The model under review builds one solid part; all positions refer to its coordinate system, in mm. Face numbers are marked on the shaded views. A direction names the side the tool comes from. Round coordinates to 2 decimals unless told otherwise and drop trailing zeros. Write each loop counter-clockwise with the first axis right and the second up, starting at its lowest first coordinate (ties: lowest second). Pieces come first, ordered by that corner, then holes. Notation, with made-up numbers: (57, 37) -> (96, 37) arc R16 cw to (96, 43) -> close; hole circle Ø11 at (-30.75, 77.5). An arc over 180 degrees is marked (long way). Return JSON: item names as keys, results as strings. Group by question number.
1. Take a section at D-D, the plane z = 9.5. Write out the cut boundary in (x, y).
2. Take a section at A-A, the plane z = -9.75. Write out the cut boundary in (x, y).
3. Take a section at C-C, the plane x = -11.5. Give the number of separate pieces and of enclosed holes in the cut face, then the cut area to 3 significant figures.
4. For line 1 along Z through (x, y) = (-5.5, -14.5); line 2 along Z through (x, y) = (-6, 1.5); line 3 along X through (y, z) = (-8, 9), list the stretches that pass through material, from the lowest coordinate up. Write a range as from..to.
5. Take a section at B-B, the plane y = 6.5. Write out the cut boundary in (x, z), then the cut area to 3 significant figures.
6. Clearance check with flat-ended pins moving along their axes: P1, Ø4, axis at x = -25.5, y = 0.5, coming from the -Z side; P2, Ø4.5, axis at x = -4.5, y = -7.5, coming from the -Z side; P3, Ø3, axis at y = 12, z = 6.5, coming from the +X side. State where each tip first meets the part, or that it passes through.
7. Mouldability with a two-part tool opening along Y and no side actions: class the marked faces 4, 5 and 6 as pulls with the +Y half, pulls with the -Y half, needs draft (parallel to the pull), parting line crosses it, or undercut.
8. Tool access review of the marked faces 1, 2 and 3: name each direction out of +Z, -Z, +X, -X, +Y, -Y from which nothing blocks a thin tool from reaching the whole face with its end or side.
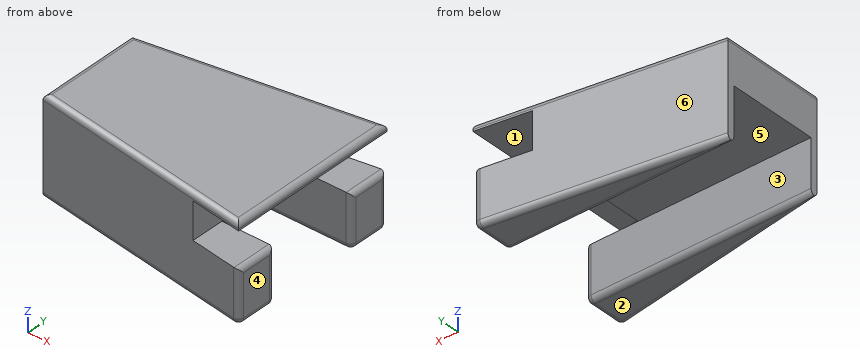
from build123d import *

# Parameters (mm, degrees)
F0_W         = 64.5
F0_H         = 13
F0_H_2       = 2
F1_DEPTH     = 12.5
F2_DEPTH     = 15
F4_DEPTH     = 15
F6_T1_DEPTH  = 72.7705906209
F6_T3_DEPTH  = 57.5
F6_T5_DEPTH  = 72.7705906209
F6_T7_DEPTH  = 37.5
F6_T9_DEPTH  = 66.75
F6_T11_DEPTH = 67.2701117692
F6_T13_DEPTH = 8.7495211484
F6_T15_DEPTH = 67.2701117692
F6_T17_DEPTH = 8.7495211484
F6_T19_DEPTH = 17.8761971291
F6_T21_DEPTH = 17.25
F6_T23_DEPTH = 19.5
F6_T25_DEPTH = 19.5
F6_S29_W     = 1.53
F6_S29_H     = 1.53
F6_T30_DEPTH = 1.53
F6_T36_DEPTH = 1.53
F6_S41_W     = 1.53
F6_S41_H     = 1.53
F6_T42_DEPTH = 1.53
F6_T48_DEPTH = 1.53
F6_T54_DEPTH = 9.5
F6_S55_R     = 1.5
F6_T56_DEPTH = 6
F6_T60_DEPTH = 9.5
F6_S61_R     = 1.5
F6_T62_DEPTH = 6
F6_T66_DEPTH = 9.5
F6_S67_R     = 1.5
F6_T68_DEPTH = 6
F6_T72_DEPTH = 9.5
F6_S73_R     = 1.5
F6_T74_DEPTH = 6


# Not quite as in the source:
# - a fillet or chamfer that OpenCascade refuses, or shapes differently, is made with other operations: its cross-section is extruded or revolved along the edge and cut away or added
# - a feature names something its author has since deleted; it is built from what else it names


with BuildPart() as f1:
    # F0 (on Top) → F1 (new body)
    with BuildSketch(Plane.XY):
        with Locations((-32.25, -6.5)):
            Rectangle(F0_W, F0_H)
        with Locations((-32.25, -14)):
            Rectangle(F0_W, F0_H_2)
        Polygon((0, -15), (-64.5, -15), (0, -25), align=None)
    extrude(amount=F1_DEPTH)

    # F0 (on Top) → F2 (join)
    with BuildSketch(Plane.XY):
        with Locations((-32.25, -14)):
            Rectangle(F0_W, F0_H_2)
        Polygon((0, -15), (-64.5, -15), (0, -25), align=None)
    extrude(amount=-F2_DEPTH)

    # F3 (on face) → F4 (cut)
    with BuildSketch(Plane.YZ):
        Polygon((-13, 0), (0, 0), (0, 10.5), (-25, 10.5), (-25, 0), align=None)
    extrude(amount=-F4_DEPTH, mode=Mode.SUBTRACT)

    # F5: F1 across plane


with BuildPart() as f1_1:
    add(f1.part)
    add(f1.part.mirror(Plane.XZ))

    # F6: fillet of radius 1.5 on 18 edges, made by hand

    # F6_s2 → F6_t1 (cut)
    with BuildSketch(Plane(origin=(-64.4207380098, 9.9877113194, 0), x_dir=(0, 0, 1), z_dir=(0.9881939076, -0.1532083578, 0))):
        with BuildLine():
            ThreePointArc((11, 24.7048476911), (12.0606601718, 24.2655078629), (12.5, 23.2048476911))
            Line((12.5, 23.2048476911), (12.5, 24.7048476911))
            Line((12.5, 24.7048476911), (11, 24.7048476911))
        make_face()
    extrude(amount=F6_T1_DEPTH, mode=Mode.SUBTRACT)

    # F6_s4 → F6_t3 (cut)
    with BuildSketch(Plane.XZ.offset(-28.75)):
        with BuildLine():
            ThreePointArc((-1.5, 12.5), (-0.4393398282, 12.0606601718), (0, 11))
            Line((0, 11), (0, 12.5))
            Line((0, 12.5), (-1.5, 12.5))
        make_face()
    extrude(amount=F6_T3_DEPTH, mode=Mode.SUBTRACT)

    # F6_s6 → F6_t5 (cut)
    with BuildSketch(Plane(origin=(-64.4207380098, -9.9877113194, 0), x_dir=(0, 0, 1), z_dir=(0.9881939076, 0.1532083578, 0))):
        with BuildLine():
            ThreePointArc((12.5, -23.2048476911), (12.0606601718, -24.2655078629), (11, -24.7048476911))
            Line((11, -24.7048476911), (12.5, -24.7048476911))
            Line((12.5, -24.7048476911), (12.5, -23.2048476911))
        make_face()
    extrude(amount=F6_T5_DEPTH, mode=Mode.SUBTRACT)

    # F6_s8 → F6_t7 (cut)
    with BuildSketch(Plane.XZ.offset(-18.75)):
        with BuildLine():
            ThreePointArc((-63, 12.5), (-64.0606601718, 12.0606601718), (-64.5, 11))
            Line((-64.5, 11), (-64.5, 12.5))
            Line((-64.5, 12.5), (-63, 12.5))
        make_face()
    extrude(amount=F6_T7_DEPTH, mode=Mode.SUBTRACT)

    # F6_s10 → F6_t9 (cut)
    with BuildSketch(Plane.YZ.offset(-68.25)):
        with BuildLine():
            ThreePointArc((-13, -13.5), (-13.4393398282, -14.5606601718), (-14.5, -15))
            Line((-14.5, -15), (-13, -15))
            Line((-13, -15), (-13, -13.5))
        make_face()
        with BuildLine():
            ThreePointArc((13, -13.5), (13.4393398282, -14.5606601718), (14.5, -15))
            Line((14.5, -15), (13, -15))
            Line((13, -15), (13, -13.5))
        make_face()
    extrude(amount=F6_T9_DEPTH, mode=Mode.SUBTRACT)

    # F6_s12 → F6_t11 (cut)
    with BuildSketch(Plane(origin=(-64.4207380098, 9.9877113194, 0), x_dir=(0, 0, 1), z_dir=(0.9881939076, -0.1532083578, 0))):
        with BuildLine():
            ThreePointArc((-13.5, 24.7048476911), (-14.5606601718, 24.2655078629), (-15, 23.2048476911))
            Line((-15, 23.2048476911), (-15, 24.7048476911))
            Line((-15, 24.7048476911), (-13.5, 24.7048476911))
        make_face()
    extrude(amount=F6_T11_DEPTH, mode=Mode.SUBTRACT)

    # F6_s14 → F6_t13 (cut)
    with BuildSketch(Plane.XZ.offset(14.5)):
        with BuildLine():
            ThreePointArc((0, -13.5), (-0.4393398282, -14.5606601718), (-1.5, -15))
            Line((-1.5, -15), (0, -15))
            Line((0, -15), (0, -13.5))
        make_face()
    extrude(amount=F6_T13_DEPTH, mode=Mode.SUBTRACT)

    # F6_s16 → F6_t15 (cut)
    with BuildSketch(Plane(origin=(-64.4207380098, -9.9877113194, 0), x_dir=(0, 0, 1), z_dir=(0.9881939076, 0.1532083578, 0))):
        with BuildLine():
            ThreePointArc((-15, -23.2048476911), (-14.5606601718, -24.2655078629), (-13.5, -24.7048476911))
            Line((-13.5, -24.7048476911), (-15, -24.7048476911))
            Line((-15, -24.7048476911), (-15, -23.2048476911))
        make_face()
    extrude(amount=F6_T15_DEPTH, mode=Mode.SUBTRACT)

    # F6_s18 → F6_t17 (cut)
    with BuildSketch(Plane.XZ.offset(-23.2495211484)):
        with BuildLine():
            ThreePointArc((-1.5, -15), (-0.4393398282, -14.5606601718), (0, -13.5))
            Line((0, -13.5), (0, -15))
            Line((0, -15), (-1.5, -15))
        make_face()
    extrude(amount=F6_T17_DEPTH, mode=Mode.SUBTRACT)

    # F6_s20 → F6_t19 (cut)
    with BuildSketch(Plane.XY.offset(-13.5)):
        with BuildLine():
            ThreePointArc((-1.7298125367, -24.7318120098), (-0.5239669076, -24.3885380062), (0, -23.2495211484))
            Line((0, -23.2495211484), (0, -25))
            Line((0, -25), (-1.7298125367, -24.7318120098))
        make_face()
        with BuildLine():
            ThreePointArc((0, 23.2495211484), (-0.5239669076, 24.3885380062), (-1.7298125367, 24.7318120098))
            Line((-1.7298125367, 24.7318120098), (0, 25))
            Line((0, 25), (0, 23.2495211484))
        make_face()
    extrude(amount=F6_T19_DEPTH, mode=Mode.SUBTRACT)

    # F6_s22 → F6_t21 (cut)
    with BuildSketch(Plane.XY.offset(-13.5)):
        with BuildLine():
            ThreePointArc((-1.5, -13), (-0.4393398282, -13.4393398282), (0, -14.5))
            Line((0, -14.5), (0, -13))
            Line((0, -13), (-1.5, -13))
        make_face()
        with BuildLine():
            ThreePointArc((-1.5, 13), (-0.4393398282, 13.4393398282), (0, 14.5))
            Line((0, 14.5), (0, 13))
            Line((0, 13), (-1.5, 13))
        make_face()
    extrude(amount=F6_T21_DEPTH, mode=Mode.SUBTRACT)

    # F6_s24 → F6_t23 (cut)
    with BuildSketch(Plane.XZ.offset(9.25)):
        with BuildLine():
            ThreePointArc((-1.5, 0), (-0.4393398282, -0.4393398282), (0, -1.5))
            Line((0, -1.5), (0, 0))
            Line((0, 0), (-1.5, 0))
        make_face()
    extrude(amount=F6_T23_DEPTH, mode=Mode.SUBTRACT)

    # F6_s26 → F6_t25 (cut)
    with BuildSketch(Plane.XZ.offset(-28.75)):
        with BuildLine():
            ThreePointArc((-1.5, 0), (-0.4393398282, -0.4393398282), (0, -1.5))
            Line((0, -1.5), (0, 0))
            Line((0, 0), (-1.5, 0))
        make_face()
    extrude(amount=F6_T25_DEPTH, mode=Mode.SUBTRACT)


with BuildPart() as f6_tool28:
    # F6_s29 → F6_t30 (new body)
    with BuildSketch(Plane.YZ.offset(-1.5)):
        with Locations((-13.735, -14.265)):
            Rectangle(F6_S29_W, F6_S29_H)
    extrude(amount=F6_T30_DEPTH)

    # F6_s31 → F6_t32 (revolve, cut)
    with BuildSketch(Plane(origin=(-1.5, -14.5, -13.5), x_dir=(0, -0.7071067812, 0.7071067812), z_dir=(0, 0.7071067812, 0.7071067812))):
        with BuildLine():
            ThreePointArc((0, -1.5), (1.5, 0), (0, 1.5))
            Line((0, 1.5), (0, -1.5))
        make_face()
    revolve(axis=Axis((-1.5, -14.5, -13.5), (1, 0, 0)), mode=Mode.SUBTRACT)


with BuildPart() as f1_2:
    add(f1_1.part)

    # F6_t27: cut F6_tool28
    add(f6_tool28.part, mode=Mode.SUBTRACT)


with BuildPart() as f6_tool34:
    # F6_s35 → F6_t36 (new body)
    with BuildSketch(Plane.XY.offset(-13.5)):
        Polygon((-1.5, -23.2495211484), (-1.7344087874, -24.761457827), (0.03, -25.035009577), (0.03, -23.2495211484), align=None)
    extrude(amount=-F6_T36_DEPTH)

    # F6_s37 → F6_t38 (revolve, cut)
    with BuildSketch(Plane(origin=(-1.5, -23.2495211484, -13.5), x_dir=(-0.6506887283, 0.7593445719, 0), z_dir=(-0.7593445719, -0.6506887283, 0))):
        with BuildLine():
            ThreePointArc((0, -1.5), (1.5, 0), (0, 1.5))
            Line((0, 1.5), (0, -1.5))
        make_face()
    revolve(axis=Axis((-1.5, -23.2495211484, -13.5), (0, 0, -1)), mode=Mode.SUBTRACT)


with BuildPart() as f1_3:
    add(f1_2.part)

    # F6_t33: cut F6_tool34
    add(f6_tool34.part, mode=Mode.SUBTRACT)


with BuildPart() as f6_tool40:
    # F6_s41 → F6_t42 (new body)
    with BuildSketch(Plane.YZ.offset(-1.5)):
        with Locations((13.735, -14.265)):
            Rectangle(F6_S41_W, F6_S41_H)
    extrude(amount=F6_T42_DEPTH)

    # F6_s43 → F6_t44 (revolve, cut)
    with BuildSketch(Plane(origin=(-1.5, 14.5, -13.5), x_dir=(0, 0.7071067812, 0.7071067812), z_dir=(0, 0.7071067812, -0.7071067812))):
        with BuildLine():
            ThreePointArc((0, -1.5), (1.5, 0), (0, 1.5))
            Line((0, 1.5), (0, -1.5))
        make_face()
    revolve(axis=Axis((-1.5, 14.5, -13.5), (1, 0, 0)), mode=Mode.SUBTRACT)


with BuildPart() as f1_4:
    add(f1_3.part)

    # F6_t39: cut F6_tool40
    add(f6_tool40.part, mode=Mode.SUBTRACT)


with BuildPart() as f6_tool46:
    # F6_s47 → F6_t48 (new body)
    with BuildSketch(Plane.XY.offset(-13.5)):
        Polygon((-1.5, 23.2495211484), (0.03, 23.2495211484), (0.03, 25.035009577), (-1.7344087874, 24.761457827), align=None)
    extrude(amount=-F6_T48_DEPTH)

    # F6_s49 → F6_t50 (revolve, cut)
    with BuildSketch(Plane(origin=(-1.5, 23.2495211484, -13.5), x_dir=(-0.6506887283, -0.7593445719, 0), z_dir=(0.7593445719, -0.6506887283, 0))):
        with BuildLine():
            ThreePointArc((0, -1.5), (1.5, 0), (0, 1.5))
            Line((0, 1.5), (0, -1.5))
        make_face()
    revolve(axis=Axis((-1.5, 23.2495211484, -13.5), (0, 0, -1)), mode=Mode.SUBTRACT)


with BuildPart() as f1_5:
    add(f1_4.part)

    # F6_t45: cut F6_tool46
    add(f6_tool46.part, mode=Mode.SUBTRACT)


with BuildPart() as f6_tool52:
    # F6_s53 → F6_t54 (new body)
    with BuildSketch(Plane.XZ.offset(9.25)):
        with BuildLine():
            ThreePointArc((-63, -15), (-64.0606601718, -14.5606601718), (-64.5, -13.5))
            Line((-64.5, -13.5), (-64.5, -15))
            Line((-64.5, -15), (-63, -15))
        make_face()
    extrude(amount=F6_T54_DEPTH)

    # F6_s55 → F6_t56 (cut, symmetric)
    with BuildSketch(Plane(origin=(-60.1810089756, 9.3303889885, 0), x_dir=(0, 0, 1), z_dir=(-0.9881939076, 0.1532083578, 0))):
        with Locations((-13.5, -23.2048476911)):
            Circle(F6_S55_R)
    extrude(amount=F6_T56_DEPTH, both=True, mode=Mode.SUBTRACT)


with BuildPart() as f1_6:
    add(f1_5.part)

    # F6_t51: cut F6_tool52
    add(f6_tool52.part, mode=Mode.SUBTRACT)


with BuildPart() as f6_tool58:
    # F6_s59 → F6_t60 (new body)
    with BuildSketch(Plane.XZ.offset(9.25)):
        with BuildLine():
            ThreePointArc((-63, -15), (-64.0606601718, -14.5606601718), (-64.5, -13.5))
            Line((-64.5, -13.5), (-64.5, -15))
            Line((-64.5, -15), (-63, -15))
        make_face()
    extrude(amount=F6_T60_DEPTH)

    # F6_s61 → F6_t62 (cut, symmetric)
    with BuildSketch(Plane.YZ.offset(-63.8)):
        with Locations((-14.5, -13.5)):
            Circle(F6_S61_R)
    extrude(amount=F6_T62_DEPTH, both=True, mode=Mode.SUBTRACT)


with BuildPart() as f1_7:
    add(f1_6.part)

    # F6_t57: cut F6_tool58
    add(f6_tool58.part, mode=Mode.SUBTRACT)


with BuildPart() as f6_tool64:
    # F6_s65 → F6_t66 (new body)
    with BuildSketch(Plane.XZ.offset(-9.25)):
        with BuildLine():
            ThreePointArc((-63, -15), (-64.0606601718, -14.5606601718), (-64.5, -13.5))
            Line((-64.5, -13.5), (-64.5, -15))
            Line((-64.5, -15), (-63, -15))
        make_face()
    extrude(amount=-F6_T66_DEPTH)

    # F6_s67 → F6_t68 (cut, symmetric)
    with BuildSketch(Plane(origin=(-60.1810089756, -9.3303889885, 0), x_dir=(0, 0, 1), z_dir=(-0.9881939076, -0.1532083578, 0))):
        with Locations((-13.5, 23.2048476911)):
            Circle(F6_S67_R)
    extrude(amount=F6_T68_DEPTH, both=True, mode=Mode.SUBTRACT)


with BuildPart() as f1_8:
    add(f1_7.part)

    # F6_t63: cut F6_tool64
    add(f6_tool64.part, mode=Mode.SUBTRACT)


with BuildPart() as f6_tool70:
    # F6_s71 → F6_t72 (new body)
    with BuildSketch(Plane.XZ.offset(-9.25)):
        with BuildLine():
            ThreePointArc((-63, -15), (-64.0606601718, -14.5606601718), (-64.5, -13.5))
            Line((-64.5, -13.5), (-64.5, -15))
            Line((-64.5, -15), (-63, -15))
        make_face()
    extrude(amount=-F6_T72_DEPTH)

    # F6_s73 → F6_t74 (cut, symmetric)
    with BuildSketch(Plane.YZ.offset(-63.8)):
        with Locations((14.5, -13.5)):
            Circle(F6_S73_R)
    extrude(amount=F6_T74_DEPTH, both=True, mode=Mode.SUBTRACT)


with BuildPart() as f1_9:
    add(f1_8.part)

    # F6_t69: cut F6_tool70
    add(f6_tool70.part, mode=Mode.SUBTRACT)


solid = f1_9.part
Output:
{
 "1": {"outline": "(-64.5, -15) -> (-15, -22.67) -> (-15, 22.67) -> (-64.5, 15) -> close"},
 "2": {"outline": "(-64.5, -15) -> (-1.73, -24.73) arc R1.5 ccw to (0, -23.25) -> (0, -14.5) arc R1.5 ccw to (-1.5, -13) -> (-64.5, -13) -> close; (-64.5, 13) -> (-1.5, 13) arc R1.5 ccw to (0, 14.5) -> (0, 23.25) arc R1.5 ccw to (-1.73, 24.73) -> (-64.5, 15) -> close"},
 "3": {"separate pieces": "3", "enclosed holes": "0", "area": "396 mm^2"},
 "4": {"line 1": "z = -15..0, 10.5..12.5", "line 2": "z = 10.5..12.5", "line 3": "x = -64.5..-15"},
 "5": {"outline": "(-64.5, 0) -> (-15, 0) -> (-15, 10.5) -> (0, 10.5) -> (0, 11) arc R1.5 ccw to (-1.5, 12.5) -> (-63, 12.5) arc R1.5 ccw to (-64.5, 11) -> close", "area": "648 mm^2"},
 "6": {"P1": "stops at z = 0", "P2": "stops at z = 10.5", "P3": "stops at x = -15"},
 "7": {"face 4": "needs draft", "face 5": "undercut", "face 6": "pulls with the +Y half"},
 "8": {"face 1": "+X, +Y, -Y", "face 2": "-Z, +X, -X, +Y, -Y", "face 3": "-Z, +X, -X"}
}
